Verification items for the finished model (mm, model axes). A direction names the side the tool comes from. Give positions to 0.01 mm unless a question says otherwise; leave off trailing zeros. Loops run counter-clockwise (first coordinate to the right, second up) from the corner with the lowest first, then second, coordinate; pieces in that order, holes last. Notation, with made-up numbers: (77.5, 48) - (108.5, 48) arc R24 ccw to (108.5, 66) - close; hole circle Ø7 at (9.5, 58.5). An arc over 180 degrees is marked (long way). One line per item, written item: value. Start each with the question number.
1. Sectioned sample at D-D (z = -28.5). Record the cut outline in (x, y), plus the area to 3 significant figures.
2. Gauge pin test, flat ends, axial feed: pin 1 (4 mm diameter, centred on x = 36.5, y = 17.5, fed in from +Z); pin 2 (1.5 mm diameter, centred on y = 24, z = 38.5, fed in from -X); pin 3 (7.5 mm diameter, centred on x = 43, y = 7, fed in from -Z); pin 4 (12 mm diameter, centred on x = 45, y = 6.5, fed in from +Z). Record the tip position at first contact, or that the pin passes through.
3. Sectioned sample at B-B (z = 0). Record the cut outline in (x, y), plus the area to 3 significant figures.
4. Mould release check, pull along X, two halves, no side actions. Record for faces 5 (the flat face through (0, 10, 60)), 6 (the flat face through (-10, -23, 1)), 7 (the cylindrical face through (20, 10, 0)): pulls with the +X half, pulls with the -X half, needs draft (parallel to the pull), parting line crosses it, or undercut.
5. Scan lines: L1, parallel to X at y = 71, z = 4; L2, parallel to Y at x = -25, z = 19; L3, parallel to Z at x = 9, y = 21. Record each from-to range of solid material in increasing order. Write a range as [from, to].
6. Access from +Z, -Z, +X, -X, +Y, -Y to the whole of each face (thin tool, end or side, straight path). Record for faces 1 (the flat face through (-29, 20, -14)), 2 (the flat face through (28, 0, -14)), 3 (the flat face through (-42, 10, 15)), 4 (the flat face through (10, 44, 1)).
7. Sectioned sample at C-C (x = 46.5). Record the cut outline in (y, z).
8. Sectioned sample at A-A (y = 10). Record the cut outline in (x, z).
from build123d import *

# Parameters (mm, degrees)
CROQUIS1_W              = 150
CROQUIS1_H              = 120
SALIENTE_EXTRUIR1_DEPTH = 20
REDONDEO1_R             = 40
SALIENTE_EXTRUIR3_DEPTH = 10
CORTAR_EXTRUIR1_DEPTH   = 33.5


with BuildPart() as part:
    # Croquis1 → Saliente-Extruir1 (new body)
    with BuildSketch(Plane(origin=(0, 0, 0), x_dir=(1, 0, 0), z_dir=(0, 1, 0))):
        Rectangle(CROQUIS1_W, CROQUIS1_H)
    extrude(amount=SALIENTE_EXTRUIR1_DEPTH)

    # Redondeo1
    redondeo1_edges = [part.edges().sort_by_distance(p)[0] for p in [
        (-75, 10, -60),
        (75, 10, -60),
        (75, 10, 60),
        (-75, 10, 60),
    ]]
    fillet(redondeo1_edges, radius=REDONDEO1_R)

    # Croquis3 → Saliente-Extruir3 (add, symmetric)
    with BuildSketch(Plane(origin=(0, 0, 0), x_dir=(0, 0, -1), z_dir=(1, 0, 0))):
        with BuildLine():
            Line((-60, 20), (60, 20))
            ThreePointArc((60, 20), (0, 80), (-60, 20))
        make_face()
        with BuildLine():
            Line((60, 0), (-60, 0))
            ThreePointArc((-60, 0), (0, -60), (60, 0))
        make_face()
    extrude(amount=SALIENTE_EXTRUIR3_DEPTH, both=True)

    # Croquis4 → Cortar-Extruir1 (cut, symmetric)
    with BuildSketch(Plane(origin=(0, 20, 0), x_dir=(1, 0, 0), z_dir=(0, 1, 0))):
        with BuildLine():
            Line((-50, 15), (-35, 15))
            ThreePointArc((-35, 15), (-20, 0), (-35, -15))
            Line((-35, -15), (-50, -15))
            ThreePointArc((-50, -15), (-65, 0), (-50, 15))
        make_face()
        with BuildLine():
            Line((50, -15), (35, -15))
            ThreePointArc((35, -15), (20, 0), (35, 15))
            Line((35, 15), (50, 15))
            ThreePointArc((50, 15), (65, 0), (50, -15))
        make_face()
    extrude(amount=CORTAR_EXTRUIR1_DEPTH, both=True, mode=Mode.SUBTRACT)


solid = part.part
Results are:
1. outline: (-74.09, 0) - (-10, 0) - (-10, -52.8) - (10, -52.8) - (10, 0) - (74.09, 0) - (74.09, 20) - (10, 20) - (10, 72.8) - (-10, 72.8) - (-10, 20) - (-74.09, 20) - close
1. area: 5,080 mm^2
2. pin 1: stops at z = 60
2. pin 2: stops at x = -10
2. pin 3: stops at z = -59.77
2. pin 4: stops at z = 59.8
3. outline: (-75, 0) - (-65, 0) - (-65, 20) - (-75, 20) - close; (-20, 0) - (-10, 0) - (-10, -60) - (10, -60) - (10, 0) - (20, 0) - (20, 20) - (10, 20) - (10, 80) - (-10, 80) - (-10, 20) - (-20, 20) - close; (65, 0) - (75, 0) - (75, 20) - (65, 20) - close
3. area: 3,600 mm^2
4. face 5: needs draft
4. face 6: pulls with the -X half
4. face 7: undercut
5. L1: x = [-10, 10]
5. L2: y = [0, 20]
5. L3: z = [-59.99, 59.99]
6. face 1: +Z, -Z, -X, +Y
6. face 2: +Z, -Z, +X, -Y
6. face 3: +Y, -Y
6. face 4: +Z, -Z, +X, +Y
7. outline: (0, -58.31) - (20, -58.31) - (20, -15) - (0, -15) - close; (0, 15) - (20, 15) - (20, 58.31) - (0, 58.31) - close
8. outline: (-75, -20) arc R40 ccw to (-35, -60) - (35, -60) arc R40 ccw to (75, -20) - (75, 20) arc R40 ccw to (35, 60) - (-35, 60) arc R40 ccw to (-75, 20) - close; hole (-50, -15) - (-35, -15) arc R15 ccw to (-35, 15) - (-50, 15) arc R15 ccw to start; hole (35, -15) - (50, -15) arc R15 ccw to (50, 15) - (35, 15) arc R15 ccw to start
